Autodesk Inventor part; units mm, degrees
ref_plane "YZ Plane" through (0, 0, 0) normal (1, 0, 0) x (0, 1, 0)
ref_plane "XZ Plane" through (0, 0, 0) normal (0, 1, 0) x (-1, 0, 0)
ref_plane "XY Plane" through (0, 0, 0) normal (0, 0, 1) x (1, 0, 0)
sketch "Sketch1" plane through (0, 0, 0) normal (0, 0, 1) x (1, 0, 0)
  line L0 (-15.875, 0) -> (-12.7, 0)
  line L1 (-12.7, 0) -> (-12.7, 22.352)
  line L2 (-9.525, 25.527) -> (9.525, 25.527)
  line L3 (12.7, 22.352) -> (12.7, 0)
  line L4 (12.7, 0) -> (15.875, 0)
  line L5 (15.875, 0) -> (15.875, 25.527)
  line L6 (12.7, 28.702) -> (-12.7, 28.702)
  line L7 (-15.875, 25.527) -> (-15.875, 0)
  arc A0 (-9.525, 25.527) -> (-12.7, 22.352) centre (-9.525, 22.352) ccw
  arc A1 (12.7, 22.352) -> (9.525, 25.527) centre (9.525, 22.352) ccw
  arc A2 (-12.7, 28.702) -> (-15.875, 25.527) centre (-12.7, 25.527) ccw
  arc A3 (15.875, 25.527) -> (12.7, 28.702) centre (12.7, 25.527) ccw
  line L8 (0, 35.2315) -> (0, -5.8719)
  point P0 (0, 0)
  dimension "d0" = 28.702
  dimension "d1" = 31.75
  dimension "d2" = 3.175
  dimension "d3" = 3.175
  dimension "d4" = 3.175
extrude "Extrusion1" add sketch "Sketch1" along normal mid plane 330.2
sketch "Sketch4" plane through (15.875, 0, 165.1) normal (1, 0, 0) x (0, 0, -1)
  line L0 (165.1, -5.7404) -> (165.1, 34.4424) construction
  line L1 (-140.335, 0) -> (842.01, 0) construction
  circle A0 centre (165.1, 12.7) radius 3.175
  point P0 (165.1, 0)
  dimension "d34" = 12.7
  dimension "d35" = 0
  dimension "d36" = 6.35
extrude "Extrusion4" cut sketch "Sketch4" against normal up to surface (31.75 mm away)
pattern_linear "Rectangular Pattern3" count 30 spacing 25.4 along (0, 0, 1) count 30 spacing 25.4 along (0, 0, -1) of "Extrusion4"
equation "\"d5\" = ExtensionLen"
equation "\"ExtensionLen\" = 330.2"
properties part number "NTowerChannelExtension" material "Aluminum 6061"
Part model, mm, in its own coordinate system. A direction names the side the tool comes from. Coordinates: 2 decimals unless noted, no trailing zeros. Write each loop counter-clockwise with the first axis right and the second up, starting at its lowest first coordinate (ties: lowest second). Pieces come first, ordered by that corner, then holes.
Item 1: Mould opens along Y. For faces 1 (the face through (-15.875, 10, -2)), 2 (the face through (14.31, 11.48, 149.47)) say: released by +Y, released by -Y, zero draft, split by the parting line, or undercut.
Item 2: Slice it at C-C (y = 12.7). Count the separate pieces of the cut face and the enclosed holes in it, and give its area (3 significant figures).
Item 3: Probe line 1 (X direction, y = 18, z = 121.5) (3 decimals); line 2 (Y direction, x = 14.8, z = -50.8) (3 decimals); line 3 (Y direction, x = 15.15, z = 0) (3 decimals). List the from-to ranges inside material, lowest first.
Item 4: Slice it at A-A (z = -152.4). Write the cut outline in (x, y) (3 decimals).
Item 5: Pin check, flat tip, straight feed: pin 1 (9.5 mm diameter, centred on x = -1.5, z = 66, fed in from -Y). Stop position of the tip, or through.
Item 6: Slice it at B-B (z = 118). Write the cut outline in (x, y) (3 decimals).
Item 7: Which spindle directions (+Z, -Z, +X, -X, +Y, -Y) get a long thin tool onto all of the face, cutting with end or side? Do faces 3 (the face through (12.7, 9, -2)), 4 (the face through (-1, 26, 165.1)). Say none if no direction does.
Item 8: Slice it at D-D (x = -2). Write the cut outline in (y, z).
Results found:
1. face 1: zero draft
1. face 2: undercut
2. separate pieces: 28
2. enclosed holes: 0
2. area: 1,570 mm2
3. line 1: x = -15.875 to -12.7, 12.7 to 15.875
3. line 2: y = 0 to 9.525, 15.875 to 27.908
3. line 3: y = 0 to 9.525, 15.875 to 27.546
4. outline: (-15.875, 0) - (-12.7, 0) - (-12.7, 9.525) - (-15.875, 9.525) - close; (-15.875, 15.875) - (-12.7, 15.875) - (-12.7, 22.352) arc R3.175 cw to (-9.525, 25.527) - (9.525, 25.527) arc R3.175 cw to (12.7, 22.352) - (12.7, 15.875) - (15.875, 15.875) - (15.875, 25.527) arc R3.175 ccw to (12.7, 28.702) - (-12.7, 28.702) arc R3.175 ccw to (-15.875, 25.527) - close; (12.7, 0) - (15.875, 0) - (15.875, 9.525) - (12.7, 9.525) - close
5. pin 1: stops at y = 25.53
6. outline: (-15.875, 0) - (-12.7, 0) - (-12.7, 22.352) arc R3.175 cw to (-9.525, 25.527) - (9.525, 25.527) arc R3.175 cw to (12.7, 22.352) - (12.7, 0) - (15.875, 0) - (15.875, 25.527) arc R3.175 ccw to (12.7, 28.702) - (-12.7, 28.702) arc R3.175 ccw to (-15.875, 25.527) - close
7. face 3: +Z, -Z, -Y
7. face 4: +Z, +X, -X, +Y, -Y
8. outline: (25.53, -165.1) - (28.7, -165.1) - (28.7, 165.1) - (25.53, 165.1) - close
